from build123d import *

# Parameters (mm, degrees)
SALIENTE_EXTRUIR1_DEPTH           = 73.717911
CORTAR_EXTRUIR1_REACH             = 8
CROQUIS3_R                        = 8.75
CORTAR_EXTRUIR1_DIRECTION_2_DEPTH = 0.4
CORTAR_EXTRUIR2_REACH             = 8
CROQUIS4_R                        = 1.6
CORTAR_EXTRUIR2_DIRECTION_2_DEPTH = 0.4
CROQUIS5_R                        = 3.25
CORTAR_EXTRUIR3_DEPTH             = 2.5


with BuildPart() as part:
    # Croquis1 → Saliente-Extruir1 (new body)
    with BuildSketch(Plane.XY):
        with BuildLine():
            Line((86.324875029, 72), (86.324875029, 9))
            Line((86.324875029, 9), (105, 9))
            add(Edge.make_bspline(
                [(105, 9), (93.439731725, 18.227197661), (92.324875029, 34)],
                knots=[0, 0, 0, 1, 1, 1], degree=2))
            Line((92.324875029, 34), (92.324875029, 72))
            Line((92.324875029, 72), (86.324875029, 72))
        make_face()
    saliente_extruir1 = extrude(amount=-SALIENTE_EXTRUIR1_DEPTH)

    # Simetr_a1: Saliente-Extruir1 across Front Plane
    add(saliente_extruir1.mirror(Plane.XY))

    # Croquis3 → Cortar-Extruir1 (cut, up to next)
    with BuildSketch(Plane(origin=(92.324875029, 0, 0), x_dir=(0, 0, -1), z_dir=(1, 0, 0)), mode=Mode.PRIVATE) as cortar_extruir1_sk1:
        with BuildLine():
            Line((33.54436172, 34), (26.45563828, 34))
            ThreePointArc((26.45563828, 34), (30, 33.25), (33.54436172, 34))
        make_face()
    cortar_extruir1_tool1 = extrude(cortar_extruir1_sk1.sketch, amount=-CORTAR_EXTRUIR1_REACH, mode=Mode.PRIVATE) & part.part
    add(cortar_extruir1_tool1.solids().sort_by_distance((92.324875, 33.69887, -30))[0], mode=Mode.SUBTRACT)
    # Croquis3 → Cortar-Extruir1 (cut, up to next)
    with BuildSketch(Plane(origin=(92.324875029, 0, 0), x_dir=(0, 0, -1), z_dir=(1, 0, 0)), mode=Mode.PRIVATE) as cortar_extruir1_sk2:
        with BuildLine():
            ThreePointArc((38.75, 42), (25.227718839, 49.334018852), (26.45563828, 34))
            Line((26.45563828, 34), (33.54436172, 34))
            ThreePointArc((33.54436172, 34), (37.334018852, 37.227718839), (38.75, 42))
        make_face()
    cortar_extruir1_tool2 = extrude(cortar_extruir1_sk2.sketch, amount=-CORTAR_EXTRUIR1_REACH, mode=Mode.PRIVATE) & part.part
    add(cortar_extruir1_tool2.solids().sort_by_distance((92.324875, 42.125274, -30))[0], mode=Mode.SUBTRACT)
    # Croquis3 → Cortar-Extruir1 (cut, up to next)
    with BuildSketch(Plane(origin=(92.324875029, 0, 0), x_dir=(0, 0, -1), z_dir=(1, 0, 0)), mode=Mode.PRIVATE) as cortar_extruir1_sk3:
        with Locations((-30, 42)):
            Circle(CROQUIS3_R)
    cortar_extruir1_tool3 = extrude(cortar_extruir1_sk3.sketch, amount=-CORTAR_EXTRUIR1_REACH, mode=Mode.PRIVATE) & part.part
    add(cortar_extruir1_tool3.solids().sort_by_distance((92.324875, 42, 30))[0], mode=Mode.SUBTRACT)

    # Croquis3 → Cortar-Extruir1 direction 2 (cut)
    with BuildSketch(Plane(origin=(92.324875029, 0, 0), x_dir=(0, 0, -1), z_dir=(1, 0, 0))):
        with BuildLine():
            Line((33.54436172, 34), (26.45563828, 34))
            ThreePointArc((26.45563828, 34), (30, 33.25), (33.54436172, 34))
        make_face()
        with BuildLine():
            ThreePointArc((38.75, 42), (25.227718839, 49.334018852), (26.45563828, 34))
            Line((26.45563828, 34), (33.54436172, 34))
            ThreePointArc((33.54436172, 34), (37.334018852, 37.227718839), (38.75, 42))
        make_face()
        with Locations((-30, 42)):
            Circle(CROQUIS3_R)
    extrude(amount=CORTAR_EXTRUIR1_DIRECTION_2_DEPTH, mode=Mode.SUBTRACT)

    # Croquis4 → Cortar-Extruir2 (cut, up to next)
    with BuildSketch(Plane(origin=(92.324875029, 0, 0), x_dir=(0, 0, -1), z_dir=(1, 0, 0)), mode=Mode.PRIVATE) as cortar_extruir2_sk1:
        with Locations((-57.761533754, 42)):
            Circle(CROQUIS4_R)
    cortar_extruir2_tool1 = extrude(cortar_extruir2_sk1.sketch, amount=-CORTAR_EXTRUIR2_REACH, mode=Mode.PRIVATE) & part.part
    add(cortar_extruir2_tool1.solids().sort_by_distance((92.324875, 42, 57.761534))[0], mode=Mode.SUBTRACT)
    # Croquis4 → Cortar-Extruir2 (cut, up to next)
    with BuildSketch(Plane(origin=(92.324875029, 0, 0), x_dir=(0, 0, -1), z_dir=(1, 0, 0)), mode=Mode.PRIVATE) as cortar_extruir2_sk2:
        with Locations((-63.761533754, 57)):
            Circle(CROQUIS4_R)
    cortar_extruir2_tool2 = extrude(cortar_extruir2_sk2.sketch, amount=-CORTAR_EXTRUIR2_REACH, mode=Mode.PRIVATE) & part.part
    add(cortar_extruir2_tool2.solids().sort_by_distance((92.324875, 57, 63.761534))[0], mode=Mode.SUBTRACT)
    # Croquis4 → Cortar-Extruir2 (cut, up to next)
    with BuildSketch(Plane(origin=(92.324875029, 0, 0), x_dir=(0, 0, -1), z_dir=(1, 0, 0)), mode=Mode.PRIVATE) as cortar_extruir2_sk3:
        with Locations((-51.761533754, 57)):
            Circle(CROQUIS4_R)
    cortar_extruir2_tool3 = extrude(cortar_extruir2_sk3.sketch, amount=-CORTAR_EXTRUIR2_REACH, mode=Mode.PRIVATE) & part.part
    add(cortar_extruir2_tool3.solids().sort_by_distance((92.324875, 57, 51.761534))[0], mode=Mode.SUBTRACT)
    # Croquis4 → Cortar-Extruir2 (cut, up to next)
    with BuildSketch(Plane(origin=(92.324875029, 0, 0), x_dir=(0, 0, -1), z_dir=(1, 0, 0)), mode=Mode.PRIVATE) as cortar_extruir2_sk4:
        with Locations((51.761533754, 57)):
            Circle(CROQUIS4_R)
    cortar_extruir2_tool4 = extrude(cortar_extruir2_sk4.sketch, amount=-CORTAR_EXTRUIR2_REACH, mode=Mode.PRIVATE) & part.part
    add(cortar_extruir2_tool4.solids().sort_by_distance((92.324875, 57, -51.761534))[0], mode=Mode.SUBTRACT)
    # Croquis4 → Cortar-Extruir2 (cut, up to next)
    with BuildSketch(Plane(origin=(92.324875029, 0, 0), x_dir=(0, 0, -1), z_dir=(1, 0, 0)), mode=Mode.PRIVATE) as cortar_extruir2_sk5:
        with Locations((63.761533754, 57)):
            Circle(CROQUIS4_R)
    cortar_extruir2_tool5 = extrude(cortar_extruir2_sk5.sketch, amount=-CORTAR_EXTRUIR2_REACH, mode=Mode.PRIVATE) & part.part
    add(cortar_extruir2_tool5.solids().sort_by_distance((92.324875, 57, -63.761534))[0], mode=Mode.SUBTRACT)
    # Croquis4 → Cortar-Extruir2 (cut, up to next)
    with BuildSketch(Plane(origin=(92.324875029, 0, 0), x_dir=(0, 0, -1), z_dir=(1, 0, 0)), mode=Mode.PRIVATE) as cortar_extruir2_sk6:
        with Locations((57.761533754, 42)):
            Circle(CROQUIS4_R)
    cortar_extruir2_tool6 = extrude(cortar_extruir2_sk6.sketch, amount=-CORTAR_EXTRUIR2_REACH, mode=Mode.PRIVATE) & part.part
    add(cortar_extruir2_tool6.solids().sort_by_distance((92.324875, 42, -57.761534))[0], mode=Mode.SUBTRACT)

    # Croquis4 → Cortar-Extruir2 direction 2 (cut)
    with BuildSketch(Plane(origin=(92.324875029, 0, 0), x_dir=(0, 0, -1), z_dir=(1, 0, 0))):
        with Locations((-57.761533754, 42)):
            Circle(CROQUIS4_R)
        with Locations((-63.761533754, 57)):
            Circle(CROQUIS4_R)
        with Locations((-51.761533754, 57)):
            Circle(CROQUIS4_R)
        with Locations((51.761533754, 57)):
            Circle(CROQUIS4_R)
        with Locations((63.761533754, 57)):
            Circle(CROQUIS4_R)
        with Locations((57.761533754, 42)):
            Circle(CROQUIS4_R)
    extrude(amount=CORTAR_EXTRUIR2_DIRECTION_2_DEPTH, mode=Mode.SUBTRACT)

    # Croquis5 → Cortar-Extruir3 (cut)
    with BuildSketch(Plane(origin=(93.124875029, 0, 0), x_dir=(0, 0, -1), z_dir=(1, 0, 0))):
        with Locations((-57.761533754, 42)):
            Circle(CROQUIS5_R)
        with Locations((-63.761533754, 57)):
            Circle(CROQUIS5_R)
        with Locations((-51.761533754, 57)):
            Circle(CROQUIS5_R)
        with Locations((51.761533754, 57)):
            Circle(CROQUIS5_R)
        with Locations((63.761533754, 57)):
            Circle(CROQUIS5_R)
        with Locations((57.761533754, 42)):
            Circle(CROQUIS5_R)
    extrude(amount=-CORTAR_EXTRUIR3_DEPTH, mode=Mode.SUBTRACT)


solid = part.part
The model under review builds one solid part; all positions refer to its coordinate system, in mm. A direction names the side the tool comes from. Coordinates: 2 decimals unless noted, no trailing zeros. Write each loop counter-clockwise with the first axis right and the second up, starting at its lowest first coordinate (ties: lowest second). Pieces come first, ordered by that corner, then holes. Notation, with made-up numbers: (71, 47) - (111, 47) arc R35 cw to (111, 79) - close; hole circle Ø3 at (-39, 23.5). An arc over 180 degrees is marked (long way). Answer as a JSON object with one key per item and string values. Group by question number.
1. Add section A-A (x = 89.25). Give the number of separate pieces and of enclosed holes in the cut face, plus the area to 3 significant figures.
2. Machinability: for faces 1 (the face through (89.4, 33.46, 31.9)), 2 (the face through (91.487, 60.222, -51.338)), which of the approach directions +Z, -Z, +X, -X, +Y, -Y give a long, thin tool a straight path to every point of the face, cutting with its end or side? Answer none if there is none.
3. Mouldability with a two-part tool opening along Z and no side actions: class faces 3 (the face through (86.325, 41, -1)), 4 (the face through (91.487, 60.222, 52.185)), 5 (the face through (91, 34, 73.718)) as pulls with the +Z half, pulls with the -Z half, needs draft (parallel to the pull), parting line crosses it, or undercut.
4. Clearance check with flat-ended pins moving along their axes: pin 1 Ø5 at (y, z) = (41.5, -59) entering from +X; pin 2 Ø2 at (y, z) = (55.5, 53) entering from +X. State where each tip first meets the part, or that it passes through.
5. To check wall thickness, follow probe 1 along Y at (x, z) = (91, -30); probe 2 along X at (y, z) = (44, 15); probe 3 along Z at (x, y) = (92, 47.5). State the ranges of each line that lie inside material, in increasing order.
6. Add section B-B (y = 47). Give the boundary of the cut face in (x, z), plus the area to 3 significant figures.
Findings:
{
 "1": {"separate pieces": "1", "enclosed holes": "8", "area": "8,760 mm²"},
 "2": {"face 1": "+X, -X", "face 2": "+X"},
 "3": {"face 3": "needs draft", "face 4": "undercut", "face 5": "pulls with the +Z half"},
 "4": {"pin 1": "x = 92.32", "pin 2": "x = 90.62"},
 "5": {"probe 1": "9 to 33.25, 50.75 to 72", "probe 2": "86.32 to 92.32", "probe 3": "-73.72 to -36.81, -23.19 to 23.19, 36.81 to 73.72"},
 "6": {"outline": "(86.32, -73.72) - (92.32, -73.72) - (92.32, -37.18) - (86.32, -37.18) - close; (86.32, -22.82) - (92.32, -22.82) - (92.32, 22.82) - (86.32, 22.82) - close; (86.32, 37.18) - (92.32, 37.18) - (92.32, 73.72) - (86.32, 73.72) - close", "area": "712 mm²"}
}
